Job drawing, mm, ordinate dimensions from the low corner. One solid piece. Give positions to 0.01 mm unless a question says otherwise; leave off trailing zeros. Order: outer loops, then holes, each group sorted by start corner. A loop starts at its lowest first (then second) coordinate and runs counter-clockwise, first axis right, second up. Notation, with made-up numbers: (77, 55.5) - (126, 55.5) arc R22 ccw to (126, 88.5) - close; hole circle Ø8 at (-23.75, -21.75). An arc over 180 degrees is marked (long way). Use one line per item in the form item = value. Start each with the question number.
1. Pin check, flat tip, straight feed: P1, Ø1, axis at x = 165, z = 32, coming from the -Y side. Stop position of the tip, or through.
2. Drill centre lines: line 1 (X direction, y = 4.55, z = 52.5); line 2 (Z direction, x = 50.5, y = 0.95); line 3 (X direction, y = 4.95, z = 56). Where is each one in solid material? Low to high.
3. Band-saw the part on A-A, the plane z = 52.5. List the corners of the cut face in (x, y), plus the area to 3 significant figures.
4. Band-saw the part on B-B, the plane y = 2.8. List the corners of the cut face in (x, z), plus the area to 3 significant figures.
5. Band-saw the part on C-C, the plane x = 80. List the corners of the cut face in (y, z).
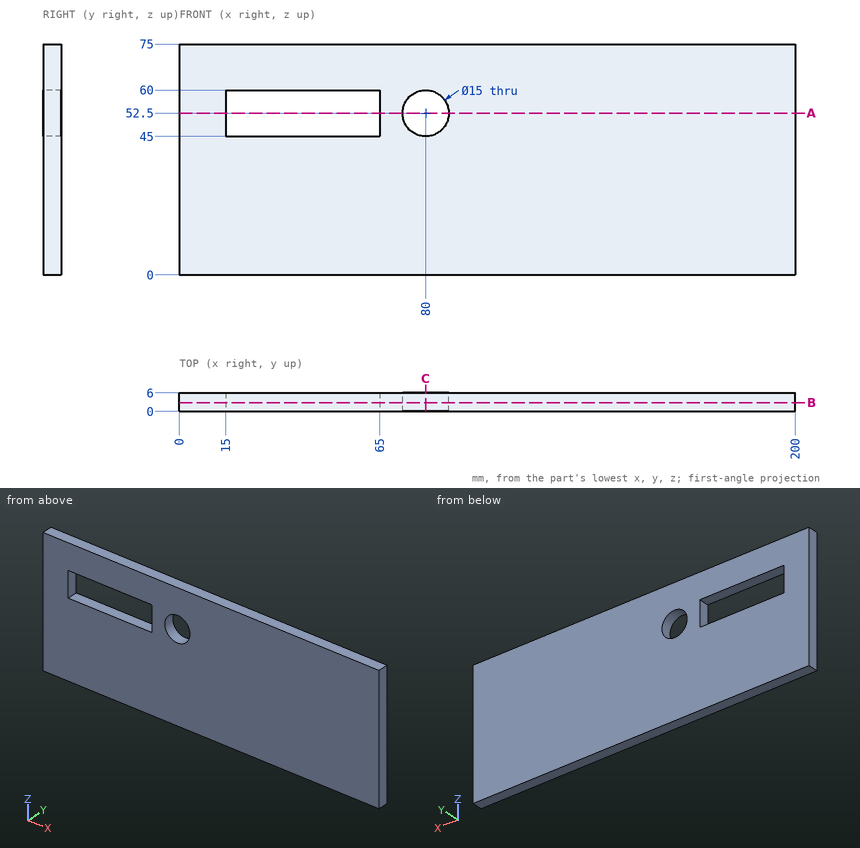
From the geometry:
q1.P1 = 0
q2.line_1 = 0 to 15, 65 to 72.5, 87.5 to 200
q2.line_2 = 0 to 45, 60 to 75
q2.line_3 = 0 to 15, 65 to 73.37, 86.63 to 200
q3.outline = (0, 0) - (15, 0) - (15, 6) - (0, 6) - close; (65, 0) - (72.5, 0) - (72.5, 6) - (65, 6) - close; (87.5, 0) - (200, 0) - (200, 6) - (87.5, 6) - close
q3.area = 810 mm²
q4.outline = (0, 0) - (200, 0) - (200, 75) - (0, 75) - close; hole (15, 45) - (65, 45) - (65, 60) - (15, 60) - close; hole circle Ø15 at (80, 52.5)
q4.area = 14,100 mm²
q5.outline = (0, 0) - (6, 0) - (6, 45) - (0, 45) - close; (0, 60) - (6, 60) - (6, 75) - (0, 75) - close
